```python
from build123d import *

# Parameters (mm, degrees)
F0_W     = 28.575
F0_H     = 6.35
F1_DEPTH = 12.7
F2_R     = 4.445
F3_DEPTH = 9.525
F4_R     = 4.445
F5_DEPTH = 9.525
F6_W     = 31.75
F6_H     = 28.575
F7_DEPTH = 9.525
F8_R     = 9.52499


# Not quite as in the source:
# - a fillet or chamfer is up to 0.001 mm smaller than in the source, because OpenCascade refuses the exact size


with BuildPart() as f1:
    # F0 (on Top) → F1 (new body)
    with BuildSketch(Plane.XY):
        with BuildLine():
            Line((-76.2, -12.7), (0, -12.7))
            Line((0, -12.7), (0, -22.225))
            Line((0, -22.225), (9.525, -22.225))
            Line((9.525, -22.225), (39.7709372272, -4.7625))
            Line((39.7709372272, -4.7625), (115.9709372272, -4.7625))
            ThreePointArc((115.9709372272, -4.7625), (124.9511933482, -8.4822438789), (128.6709372272, -17.4625))
            Line((128.6709372272, -17.4625), (166.7709372272, -17.4625))
            Line((166.7709372272, -17.4625), (166.7709372272, -7.9375))
            Line((166.7709372272, -7.9375), (192.1709372272, -7.9375))
            Line((192.1709372272, -7.9375), (192.1709372272, 7.9375))
            Line((192.1709372272, 7.9375), (166.7709372272, 7.9375))
            Line((166.7709372272, 7.9375), (166.7709372272, 17.4625))
            Line((166.7709372272, 17.4625), (128.6709372272, 17.4625))
            ThreePointArc((128.6709372272, 17.4625), (124.9511933482, 8.4822438789), (115.9709372272, 4.7625))
            Line((115.9709372272, 4.7625), (39.7709372272, 4.7625))
            Line((39.7709372272, 4.7625), (9.525, 22.225))
            Line((9.525, 22.225), (0, 22.225))
            Line((0, 22.225), (0, 12.7))
            Line((0, 12.7), (-76.2, 12.7))
            Line((-76.2, 12.7), (-76.2, -12.7))
        make_face()
        with Locations((-52.3875, 0)):
            Rectangle(F0_W, F0_H, mode=Mode.SUBTRACT)
        with Locations((-14.2875, 0)):
            Rectangle(F0_W, F0_H, mode=Mode.SUBTRACT)
    extrude(amount=F1_DEPTH)

    # F2 (on face) → F3 (join)
    with BuildSketch(Plane.XZ.offset(22.225)):
        with Locations((4.7625, 6.35)):
            Circle(F2_R)
    extrude(amount=F3_DEPTH)

    # F4 (on face) → F5 (join)
    with BuildSketch(Plane(origin=(0, 22.225, 0), x_dir=(-1, 0, 0), z_dir=(0, 1, 0))):
        with Locations((-4.7625, 6.35)):
            Circle(F4_R)
    extrude(amount=F5_DEPTH)

    # F6 (on face) → F7 (cut)
    with BuildSketch(Plane.XY.offset(12.7)):
        with Locations((147.7209372272, 0)):
            Rectangle(F6_W, F6_H)
    extrude(amount=-F7_DEPTH, mode=Mode.SUBTRACT)

    # F8 (radius 9.525 in the source; OpenCascade refuses exactly that, so slightly less here)
    f8_edges = [f1.edges().sort_by_distance(p)[0] for p in [
        (163.595937, 0, 3.175),
        (192.170937, 0, 12.7),
    ]]
    fillet(f8_edges, radius=F8_R)


solid = f1.part
```
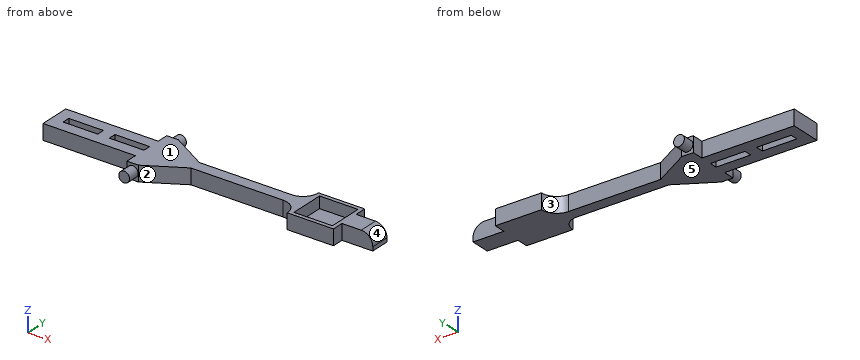
Geometry check sheet. Reference: the model listing, model coordinates, mm. Face numbers are marked on the shaded views. A direction names the side the tool comes from. Round coordinates to 2 decimals unless told otherwise and drop trailing zeros. Write each loop counter-clockwise with the first axis right and the second up, starting at its lowest first coordinate (ties: lowest second). Pieces come first, ordered by that corner, then holes. Notation, with made-up numbers: (-19, 53) - (33, 53) arc R15 ccw to (33, 72) - close; hole circle Ø4 at (34, 65.25). An arc over 180 degrees is marked (long way). Write each question's results on one line, items separated by ' | '.
(1) Set-up check for the marked faces 1 and 2: record each of +Z, -Z, +X, -X, +Y, -Y from which the full face is reachable in a straight line by a thin tool's end or side.
Computed:
face 1: +Z, +X, -X, +Y, -Y | face 2: +Z, -Z, -Y
(2) Draft check along X on the marked faces 3, 4 and 5. Enter one of: pulls with the +X half, pulls with the -X half, needs draft (parallel to the pull), parting line crosses it, or undercut.
Computed:
face 3: undercut | face 4: pulls with the +X half | face 5: needs draft
(3) Sectioned sample at C-C, the plane x = 36. Enter the section's corners in (y, z).
Computed:
outline: (-6.94, 0) - (6.94, 0) - (6.94, 12.7) - (-6.94, 12.7) - close
(4) Sectioned sample at B-B, the plane z = 6.35. Count the separate pieces of the cut face and the enclosed holes in it, plus the area to 3 significant figures.
Computed:
separate pieces: 1 | enclosed holes: 3 | area: 4,780 mm^2
(5) Depth check by flat-ended pin: pin 1 Ø6 at (y, z) = (21.5, 5) entering from -X; pin 2 Ø6.5 at (x, z) = (-18, 5) entering from -Y; pin 3 Ø5 at (y, z) = (12.5, 6.5) entering from +X; pin 4 Ø5 at (x, y) = (-19, -13) entering from -Z. Enter the tip coordinate at first touch or a pass-through.
Computed:
pin 1: stops at x = 0 | pin 2: stops at y = -12.7 | pin 3: stops at x = 166.77 | pin 4: stops at z = 0
(6) Thickness scan on probe 1 along X at (y, z) = (-9.5, 9.25); probe 2 along X at (y, z) = (-13.5, 6.25); probe 3 along Y at (x, z) = (-7, 4.75) (3 decimals). Record the ranges inside material, lowest first. Write a range as from..to.
Computed:
probe 1: x = -76.2..31.57, 125.86..131.85, 162.95..166.77 | probe 2: x = 0..24.64, 128.04..131.85, 161.08..166.77 | probe 3: y = -12.7..-3.175, 3.175..12.7
